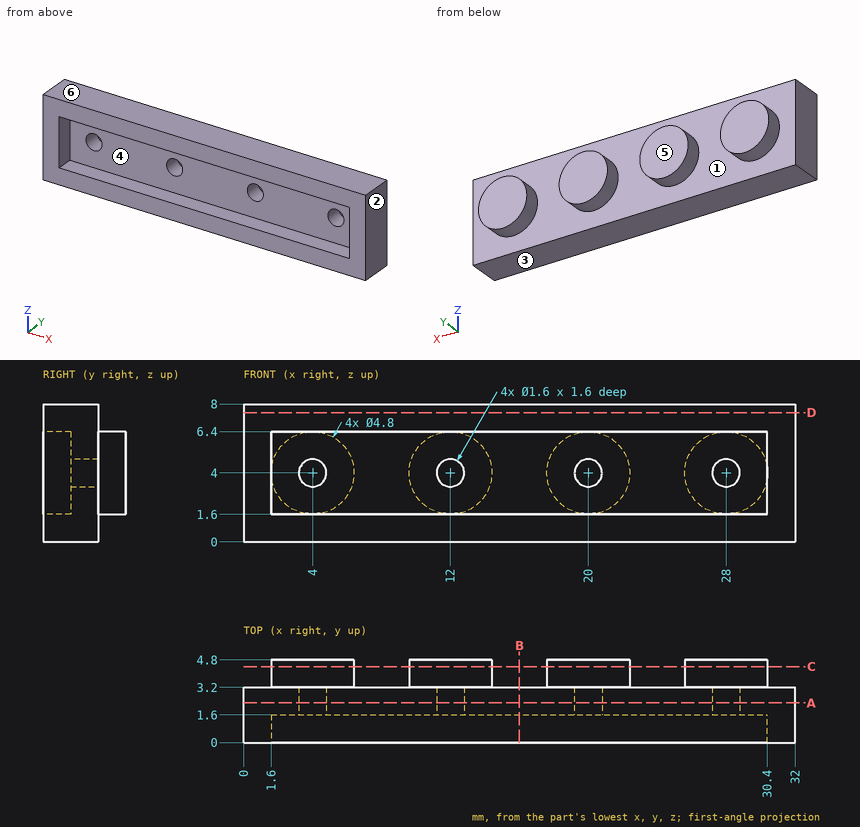
Print and shaded views of the part. All mm, measured from the part's lowest x, y and z. A direction names the side the tool comes from. Coordinates: 2 decimals unless noted, no trailing zeros. Write each loop counter-clockwise with the first axis right and the second up, starting at its lowest first coordinate (ties: lowest second). Pieces come first, ordered by that corner, then holes.
(1) Drill centre lines: probe 1 along X at (y, z) = (2.2, 4); probe 2 along X at (y, z) = (0.5, 3.5); probe 3 along Z at (x, y) = (5, 1.15). Where is each one in solid material? Low to high.
(2) Cut at A-A, the plane y = 2.3. List the corners of the cut face in (x, z), and give its area (3 significant figures).
(3) Two-plate mould, pull along Z, no slides. Class the marked faces 3, 4, 5 and 6: +Z half, -Z half, draft (parallel to the pull), parting line (faces both ways), or undercut.
(4) Cut at D-D, the plane z = 7.5. List the corners of the cut face in (x, y).
(5) 3-axis set-ups, long thin cutter, end or side, ignore diameter. For the marked faces 1 and 2: which of +Z, -Z, +X, -X, +Y, -Y reach the whole face in a straight line?
(6) Flat gauge pins, fed straight in: pin 1 (0.5 mm diameter, centred on x = 28, z = 4, fed in from -Y); pin 2 (1.8 mm diameter, centred on x = 20, z = 4.5, fed in from -Y). Where does each tip first touch, or does it go through?
(7) Cut at B-B, the plane x = 16. List the corners of the cut face in (y, z).
(8) Cut at C-C, the plane y = 4.4. List the corners of the cut face in (x, z), and give its area (3 significant figures).
Geometry says:
1. probe 1: x = 0 to 3.2, 4.8 to 11.2, 12.8 to 19.2, 20.8 to 27.2, 28.8 to 32
1. probe 2: x = 0 to 1.6, 30.4 to 32
1. probe 3: z = 0 to 1.6, 6.4 to 8
2. outline: (0, 0) - (32, 0) - (32, 8) - (0, 8) - close; hole circle Ø1.6 at (4, 4); hole circle Ø1.6 at (12, 4); hole circle Ø1.6 at (20, 4); hole circle Ø1.6 at (28, 4)
2. area: 248 mm2
3. face 3: -Z half
3. face 4: undercut
3. face 5: draft
3. face 6: +Z half
4. outline: (0, 0) - (32, 0) - (32, 3.2) - (0, 3.2) - close
5. face 1: +Y
5. face 2: +Z, -Z, +X, +Y, -Y
6. pin 1: stops at y = 3.2
6. pin 2: stops at y = 1.6
7. outline: (0, 0) - (3.2, 0) - (3.2, 8) - (0, 8) - (0, 6.4) - (1.6, 6.4) - (1.6, 1.6) - (0, 1.6) - close
8. outline: circle Ø4.8 at (4, 4); circle Ø4.8 at (12, 4); circle Ø4.8 at (20, 4); circle Ø4.8 at (28, 4)
8. area: 72.4 mm2
